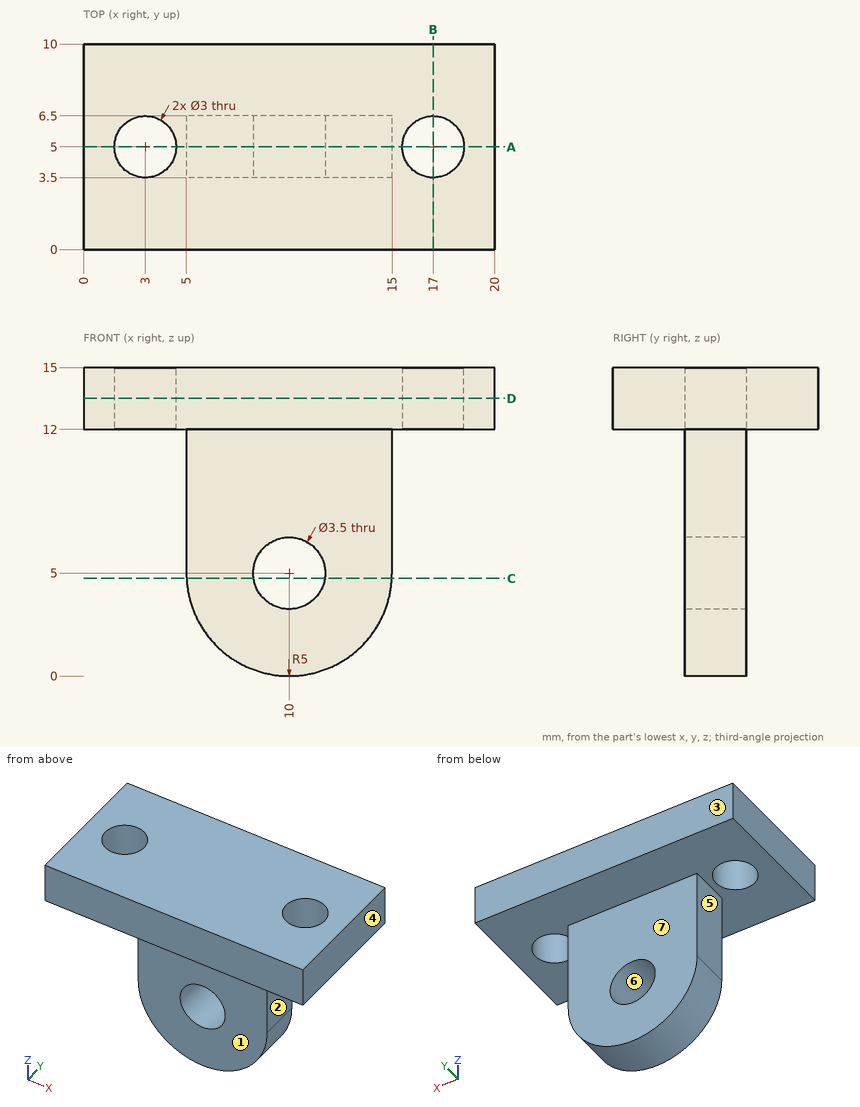
Drawing for the job (mm, zero at the part's lowest x, y, z). A direction names the side the tool comes from. Coordinates: 2 decimals unless noted, no trailing zeros. Order: outer loops, then holes, each group sorted by start corner. A loop starts at its lowest first (then second) coordinate and runs counter-clockwise, first axis right, second up. Notation, with made-up numbers: (70.5, 33.25) -> (116.5, 33.25) arc R28 cw to (116.5, 65.25) -> close; hole circle Ø2 at (77, -12.5). An arc over 180 degrees is marked (long way). Answer in a Markdown table with one row per item.
1) Band-saw the part on B-B (x = 17). List the corners of the cut face in (y, z).
Check values:
| item | result |
|---|---|
| outline | (0, 12) -> (3.5, 12) -> (3.5, 15) -> (0, 15) -> close; (6.5, 12) -> (10, 12) -> (10, 15) -> (6.5, 15) -> close |
2) Which spindle directions (+Z, -Z, +X, -X, +Y, -Y) get a long thin tool onto all of the face, cutting with end or side? Do the marked faces 1, 2 and 3. Say none if no direction does.
Check values:
| item | result |
|---|---|
| face 1 | -Z, +X, -X, -Y |
| face 2 | -Z, +X, +Y, -Y |
| face 3 | +Z, -Z, +X, -X, +Y |
3) Band-saw the part on A-A (y = 5). List the corners of the cut face in (x, z).
Check values:
| item | result |
|---|---|
| outline | (0, 12) -> (1.5, 12) -> (1.5, 15) -> (0, 15) -> close; (4.5, 12) -> (5, 12) -> (5, 5) arc R5 ccw to (15, 5) -> (15, 12) -> (15.5, 12) -> (15.5, 15) -> (4.5, 15) -> close; (18.5, 12) -> (20, 12) -> (20, 15) -> (18.5, 15) -> close; hole circle Ø3.5 at (10, 5) |
4) Band-saw the part on D-D (z = 13.5). List the corners of the cut face in (x, y).
Check values:
| item | result |
|---|---|
| outline | (0, 0) -> (20, 0) -> (20, 10) -> (0, 10) -> close; hole circle Ø3 at (3, 5); hole circle Ø3 at (17, 5) |
5) Flat gauge pins, fed straight in: P1, Ø8, axis at x = 12.5, z = 3.5, coming from the +Y side; P2, Ø2, axis at y = 3, z = 9, coming from the -X side; P3, Ø1.5, axis at y = 4.5, z = 9.5, coming from the +X side; P4, Ø1, axis at y = 1.5, z = 10, coming from the -X side. Where does each tip first touch, or does it go through?
Check values:
| item | result |
|---|---|
| P1 | y = 6.5 |
| P2 | x = 5 |
| P3 | x = 15 |
| P4 | through |
6) Mould opens along X. For the marked faces 4, 5, 6 and 7 say: pulls with the +X half, pulls with the -X half, needs draft (parallel to the pull), parting line crosses it, or undercut.
Check values:
| item | result |
|---|---|
| face 4 | pulls with the +X half |
| face 5 | pulls with the -X half |
| face 6 | undercut |
| face 7 | needs draft |
7) Band-saw the part on C-C (z = 4.75). List the corners of the cut face in (x, y), and give its area (3 significant figures).
Check values:
| item | result |
|---|---|
| outline | (5.01, 3.5) -> (8.27, 3.5) -> (8.27, 6.5) -> (5.01, 6.5) -> close; (11.73, 3.5) -> (14.99, 3.5) -> (14.99, 6.5) -> (11.73, 6.5) -> close |
| area | 19.6 mm2 |
8) Drill centre lines: line 1 (X direction, y = 5, z = 14.15); line 2 (Y direction, x = 17, z = 13.2); line 3 (Z direction, x = 10, y = 4.4). Where is each one in solid material? Low to high.
Check values:
| item | result |
|---|---|
| line 1 | 0 to 1.5, 4.5 to 15.5, 18.5 to 20 |
| line 2 | 0 to 3.5, 6.5 to 10 |
| line 3 | 0 to 3.25, 6.75 to 15 |
